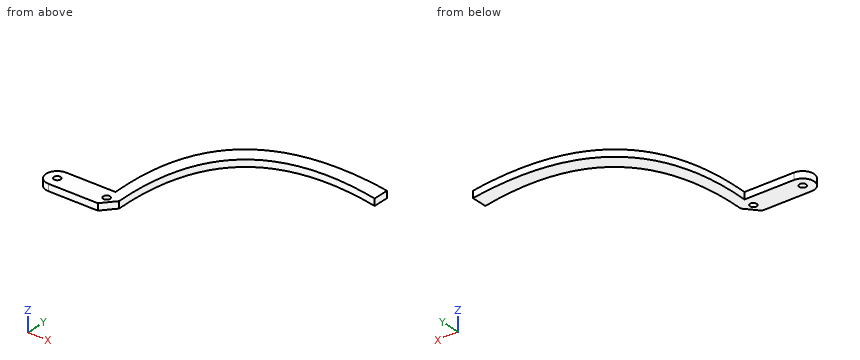
```python
from build123d import *

# Parameters (mm, degrees)
SKETCH1_R           = 1.5
BOSS_EXTRUDE1_DEPTH = 3


with BuildPart() as part:
    # Sketch1 → Boss-Extrude1 (new body)
    with BuildSketch(Plane.XY):
        with BuildLine():
            Line((0, 5), (22, 5))
            add(Edge.make_bspline(
                [(22, 5), (18.375967342, 77.940552932), (95.875501698, 64.550484918)],
                knots=[0, 0, 0, 1, 1, 1], degree=2))
            Line((95.875501698, 64.550484918), (95.875501698, 57.584409058))
            add(Edge.make_bspline(
                [(26.94328985, 0.750923068), (24.379410311, 72.075337148), (95.875501698, 57.584409058)],
                knots=[0, 0, 0, 1, 1, 1], degree=2))
            Line((26.94328985, 0.750923068), (22, -5))
            Line((22, -5), (0, -5))
            ThreePointArc((0, -5), (-5, 0), (0, 5))
        make_face()
        Circle(SKETCH1_R, mode=Mode.SUBTRACT)
        with Locations((22, 0)):
            Circle(SKETCH1_R, mode=Mode.SUBTRACT)
    extrude(amount=BOSS_EXTRUDE1_DEPTH)


solid = part.part
```
Can you work these out from the model? Positions are in its coordinate system, mm. Round coordinates to 2 decimals unless told otherwise and drop trailing zeros. Order: outer loops, then holes, each group sorted by start corner. A loop starts at its lowest first (then second) coordinate and runs counter-clockwise, first axis right, second up.
(1) If we section it at B-B (x = 12): Please give me the cut outline in (y, z).
Results are:
outline: (-5, 0) - (5, 0) - (5, 3) - (-5, 3) - close
(2) If I drill on L1, parallel to Y at x = 0, z = 2.35; L2, parallel to Y at x = 1, z = 0.4; L3, parallel to Y at x = 11.5, z = 1.15, over which ranges is the centre line in solid material (lowest first)?
Results are:
L1: y = -5 to -1.5, 1.5 to 5
L2: y = -5 to -1.12, 1.12 to 5
L3: y = -5 to 5
(3) If we section it at A-A (z = 1.15): Count the separate pieces of the cut face and the enclosed holes in it, plus the area to 3 significant figures.
Results are:
separate pieces: 1
enclosed holes: 2
area: 995 mm2
(4) I'm going to push flat-ended pins straight in: pin 1 (1.5 mm diameter, centred on x = 78.5, z = 2.5, fed in from -Y); pin 2 (5 mm diameter, centred on x = 22, y = 0, fed in from +Z); pin 3 (0.9 mm diameter, centred on x = 6.5, z = 1, fed in from +Y). Where does each tip first touch, or does it pass through?
Results are:
pin 1: stops at y = 59.86
pin 2: stops at z = 3
pin 3: stops at y = 5
